Could you check a few things on this model? Use its own coordinates, in mm. A direction names the side the tool comes from. Round coordinates to 2 decimals unless told otherwise and drop trailing zeros. Order: outer loops, then holes, each group sorted by start corner. A loop starts at its lowest first (then second) coordinate and runs counter-clockwise, first axis right, second up.
```python
from build123d import *

# Parameters (mm, degrees)
F0_W     = 1054.1
F0_H     = 990.6
F1_DEPTH = 0.762
F2_W     = 1016
F2_H     = 914.4
F3_DEPTH = 25.4
F4_R     = 1.5875
F5_DEPTH = 26.163


with BuildPart() as f1:
    # F0 (on Front) → F1 (new body)
    with BuildSketch(Plane.XZ):
        Rectangle(F0_W, F0_H)
    extrude(amount=F1_DEPTH)

    # F2 (on face) → F3 (join)
    with BuildSketch(Plane.XZ.offset(0.762)):
        with Locations((19.05, 0)):
            Rectangle(F2_W, F2_H)
    extrude(amount=F3_DEPTH)

    # F4 (on face) → F5 (cut, through all)
    with BuildSketch(Plane(origin=(0, 0, 0), x_dir=(-1, 0, 0), z_dir=(0, 1, 0))):
        with Locations((-520.7, 203.2)):
            Circle(F4_R)
        with Locations((-514.35, 222.25)):
            Circle(F4_R)
        with Locations((-514.35, 184.15)):
            Circle(F4_R)
        with Locations((-514.35, -184.15)):
            Circle(F4_R)
        with Locations((-520.7, -203.2)):
            Circle(F4_R)
        with Locations((-514.35, -222.25)):
            Circle(F4_R)
    extrude(amount=-F5_DEPTH, mode=Mode.SUBTRACT)


solid = f1.part
```
Q1. Imagine slicing it at C-C, the plane z = -116.5. Please give me the cut outline in (x, y).
Q2. I need wall thicknesses on L1, parallel to Z at x = 520.7, y = -17; L2, parallel to Z at x = 514.35, y = -19.5; L3, parallel to X at y = -9.75, z = 203.2. Which ranges of each line are inside material? Lowest first, please.
Q3. Imagine slicing it at B-B, the plane y = -14.25. State how many separate pieces and enclosed holes the cut face has, then the cut area to 3 significant figures.
Q4. For P1, Ø3, axis at x = 514.35, z = -222.25, coming from the +Y side; P2, Ø1, axis at y = -17.5, z = 5.5, coming from the -X side; P3, Ø2, axis at x = 346.5, y = -7, coming from the -Z side, each with a flat end and sliding along its axis, tell me the tip position at first contact or that it passes through.
Q5. Imagine slicing it at A-A, the plane x = 248. Please give me the cut outline in (y, z).
Q6. For faces 1 (the flat face through (-510, -0.762, 2)), 2 (the flat face through (-488.95, -13, -6)), 3 (the flat face through (12, -13, 457.2)), which set-ups out of +Z, -Z, +X, -X, +Y, -Y let a thin tool reach every point of the face, with its end or its side?
Filled in:
1. outline: (-527.05, -0.76) - (-488.95, -0.76) - (-488.95, -26.16) - (527.05, -26.16) - (527.05, 0) - (-527.05, 0) - close
2. L1: z = -457.2 to -204.79, -201.61 to 201.61, 204.79 to 457.2
2. L2: z = -457.2 to -223.84, -220.66 to -185.74, -182.56 to 182.56, 185.74 to 220.66, 223.84 to 457.2
2. L3: x = -488.95 to 519.11, 522.29 to 527.05
3. separate pieces: 1
3. enclosed holes: 6
3. area: 929,000 mm2
4. P1: passes through
4. P2: stops at x = -488.95
4. P3: stops at z = -457.2
5. outline: (-26.16, -457.2) - (-0.76, -457.2) - (-0.76, -495.3) - (0, -495.3) - (0, 495.3) - (-0.76, 495.3) - (-0.76, 457.2) - (-26.16, 457.2) - close
6. face 1: -X, -Y
6. face 2: +Z, -Z, -X, -Y
6. face 3: +Z, +X, -X, -Y
